```python
from build123d import *

# Parameters (mm, degrees)
F0_R     = 20.0378472318
F1_DEPTH = 1


with BuildPart() as f1:
    # F0 (on Top) → F1 (new body)
    with BuildSketch(Plane.XY):
        Circle(F0_R)
        with BuildLine():
            ThreePointArc((-1, -18.010106406), (-18.0377520859, 0.0585870494), (-0.8829856241, 18.0162223883))
            ThreePointArc((-0.8829856241, 18.0162223883), (0.2419860556, 18.0362239813), (1.3660161897, 17.9860482743))
            ThreePointArc((1.3660161897, 17.9860482743), (13.2288307137, 12.2622172018), (18.0378472318, 0))
            ThreePointArc((18.0378472318, 0), (13.4285198006, -12.0432050851), (1.9562398361, -17.9314544435))
            ThreePointArc((1.9562398361, -17.9314544435), (0.4797344983, -18.031466595), (-1, -18.010106406))
        make_face(mode=Mode.SUBTRACT)
        with BuildLine():
            Line((0.8829856241, 17.0774223292), (-0.8829856241, 18.0162223883))
            Line((-0.8829856241, 18.0162223883), (-10.9921143656, -1))
            Line((-10.9921143656, -1), (-1, -1))
            Line((-1, -1), (-1, -18.010106406))
            ThreePointArc((-1, -18.010106406), (0.4797344983, -18.031466595), (1.9562398361, -17.9314544435))
            Line((1.9562398361, -17.9314544435), (16.2997357547, 1))
            Line((16.2997357547, 1), (-7.6638607916, 1))
            Line((-7.6638607916, 1), (0.8829856241, 17.0774223292))
        make_face()
        Polygon((1, -15.8817395568), (1, -1), (12.2752124372, -1), align=None, mode=Mode.SUBTRACT)
        with BuildLine():
            ThreePointArc((1.3660161897, 17.9860482743), (0.2419860556, 18.0362239813), (-0.8829856241, 18.0162223883))
            Line((-0.8829856241, 18.0162223883), (0.8829856241, 17.0774223292))
            Line((0.8829856241, 17.0774223292), (1.3660161897, 17.9860482743))
        make_face()
    extrude(amount=F1_DEPTH)


solid = f1.part
```
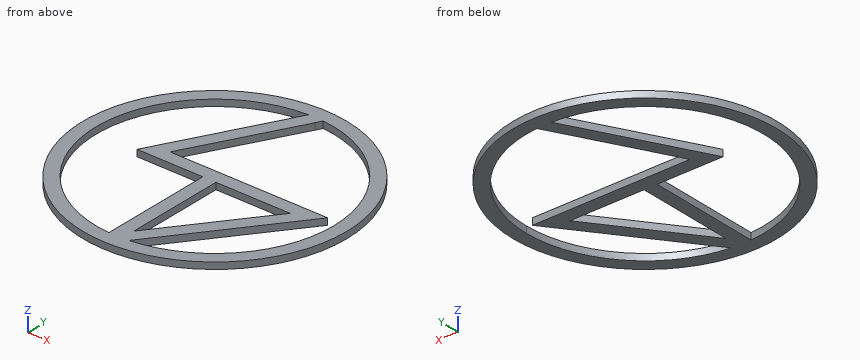
For this review, take the finished solid that the model builds, in its own axes (mm). Round coordinates to 2 decimals unless told otherwise and drop trailing zeros. Write each loop counter-clockwise with the first axis right and the second up, starting at its lowest first coordinate (ties: lowest second). Pieces come first, ordered by that corner, then holes.
1) Take a section at A-A on x = 4.5. Give the boundary of the cut face in (y, z), then the cut area to 3 significant figures.
Answer below:
outline: (-19.53, 0) - (-17.47, 0) - (-17.47, 1) - (-19.53, 1) - close; (-14.57, 0) - (-11.26, 0) - (-11.26, 1) - (-14.57, 1) - close; (-1, 0) - (1, 0) - (1, 1) - (-1, 1) - close; (17.47, 0) - (19.53, 0) - (19.53, 1) - (17.47, 1) - close
area: 9.43 mm2
2) Take a section at D-D on x = 0. Give the boundary of the cut face in (y, z), then the cut area to 3 significant figures.
Answer below:
outline: (-20.04, 0) - (1, 0) - (1, 1) - (-20.04, 1) - close; (15.42, 0) - (20.04, 0) - (20.04, 1) - (15.42, 1) - close
area: 25.7 mm2
3) Insertion check: pin 1 Ø0.5 at (x, z) = (8, 0.5) entering from +Y; pin 2 Ø10 at (x, y) = (-3, -8.5) entering from +Z. Each pin has a flat end and moves straight along its axis. Give the tip position at first contact, or say it passes through.
Answer below:
pin 1: stops at y = 18.48
pin 2: stops at z = 1
4) For line 1 along X through (y, z) = (9, 0.8); line 2 along X through (y, z) = (5, 0.85); line 3 along Y through (x, z) = (6.5, 0.1), list the stretches that pass through material, from the lowest coordinate up.
Answer below:
line 1: x = -17.9 to -15.63, -5.68 to -3.41, 15.63 to 17.9
line 2: x = -19.4 to -17.33, -7.8 to -5.54, 17.33 to 19.4
line 3: y = -18.95 to -16.83, -11.93 to -8.62, -1 to 1, 16.83 to 18.95
5) Take a section at B-B on y = -17. Give the boundary of the cut face in (x, z).
Answer below:
outline: (-10.61, 0) - (-6.03, 0) - (-6.03, 1) - (-10.61, 1) - close; (-1, 0) - (2.66, 0) - (2.66, 1) - (-1, 1) - close; (6.03, 0) - (10.61, 0) - (10.61, 1) - (6.03, 1) - close
6) Take a section at C-C on z = 0.15. Give the boundary of the cut face in (x, y), then the cut area to 3 significant figures.
Answer below:
outline: circle Ø40.08 at (0, 0); hole (-10.99, -1) - (-0.88, 18.02) arc R18.04 ccw to (-1, -18.01) - (-1, -1) - close; hole (-7.66, 1) - (16.3, 1) - (1.96, -17.93) arc R18.04 ccw to (1.37, 17.99) - close; hole (1, -15.88) - (12.28, -1) - (1, -1) - close
area: 405 mm2
